```python
from build123d import *

# Parameters (mm, degrees)
BOSS_EXTRUDE1_DEPTH = 20
SKETCH3_R           = 2.5
CUT_EXTRUDE1_DEPTH  = 101.912910248
SKETCH4_R           = 2.5
BOSS_EXTRUDE2_DEPTH = 5
SKETCH5_R           = 2.25
CUT_EXTRUDE2_DEPTH  = 101.912910248
FILLET2_R           = 2


with BuildPart() as part:
    # Sketch2 → Boss-Extrude1 (new body)
    with BuildSketch(Plane(origin=(0, 0, 0), x_dir=(1, 0, 0), z_dir=(0, 1, 0))):
        with BuildLine():
            Line((-31.365303949, 0), (78.634696051, 0))
            add(Edge.make_bspline(
                [(-31.365303949, 60), (-8.421867165, 19.05257491), (40.3762891, 8.008963313), (78.634696051, 0)],
                knots=[0, 0, 0, 0, 1, 1, 1, 1], degree=3))
            Line((-31.365303949, 60), (-31.365303949, 0))
        make_face()
    extrude(amount=BOSS_EXTRUDE1_DEPTH)

    # Sketch3 → Cut-Extrude1 (cut, through all)
    with BuildSketch(Plane.XY):
        with Locations((-11.365303949, 10)):
            Circle(SKETCH3_R)
        with Locations((8.634696051, 10)):
            Circle(SKETCH3_R)
        with Locations((28.634696051, 10)):
            Circle(SKETCH3_R)
        with Locations((48.634696051, 10)):
            Circle(SKETCH3_R)
    extrude(amount=-CUT_EXTRUDE1_DEPTH, mode=Mode.SUBTRACT)

    # Sketch4 → Boss-Extrude2 (add)
    with BuildSketch(Plane.XY):
        with Locations((-11.365303949, 10)):
            Circle(SKETCH4_R)
        with Locations((8.634696051, 10)):
            Circle(SKETCH4_R)
        with Locations((28.634696051, 10)):
            Circle(SKETCH4_R)
        with Locations((48.634696051, 10)):
            Circle(SKETCH4_R)
    extrude(amount=-BOSS_EXTRUDE2_DEPTH)

    # Sketch5 → Cut-Extrude2 (cut, through all)
    with BuildSketch(Plane.XY):
        with Locations((-11.365303949, 10)):
            Circle(SKETCH5_R)
        with Locations((8.634696051, 10)):
            Circle(SKETCH5_R)
        with Locations((28.634696051, 10)):
            Circle(SKETCH5_R)
        with Locations((48.634696051, 10)):
            Circle(SKETCH5_R)
    extrude(amount=-CUT_EXTRUDE2_DEPTH, mode=Mode.SUBTRACT)

    # Fillet2
    fillet2_edges = [part.edges().sort_by_distance(p)[0] for p in [
        (16.640660288, 20, -18.214380109),
        (16.640660288, 0, -18.214380109),
    ]]
    fillet(fillet2_edges, radius=FILLET2_R)


solid = part.part
```
Source: CAD feature listing. Evaluate the final solid. Frame: model axes, mm. A direction names the side the tool comes from. Coordinates: 2 decimals unless noted, no trailing zeros. One line per item, written item: value.
1) Reachability of faces 1 (the face through (26.137, 10.11, -9.548)), 2 (the face through (-13.024, 11.521, -2.465)) from +Z, -Z, +X, -X, +Y, -Y: full face, straight path, thin tool, end or side. Return the list, or none.
Computed values:
face 1: -Z
face 2: +Z, -Z
2) Contact query for flat-ended pins moving along their axis: pin 1 (8 mm diameter, centred on x = 53.5, y = 12.5, fed in from -Z); pin 2 (6 mm diameter, centred on x = 48.63, y = 10, fed in from -Z); pin 3 (5 mm diameter, centred on y = 8.5, z = -36, fed in from +X). Output: stop coordinate, or through.
Computed values:
pin 1: stops at z = -6.73
pin 2: stops at z = -7.8
pin 3: stops at x = -8.67
3) Ray query, line 1 (X direction, y = 10, z = -25.5); line 2 (Z direction, x = -22, y = 15); line 3 (Z direction, x = 35.5, y = 4). Return the intervals inside material, ascending. Write a range as [from, to].
Computed values:
line 1: x = [-31.37, -13.87], [-8.87, 2.83]
line 2: z = [-46.44, 0]
line 3: z = [-10.89, 0]
4) Mould query, pull axis X, two halves, no side actions, for faces 3 (the face through (-13.863, 10.11, -21.242)), 4 (the face through (-4, 0, -12)), 5 (the face through (-31.365, 10, -30)), 6 (the face through (6.976, 11.521, -2.465)). Classes: released by +X, released by -X, zero draft, split by the parting line, or undercut.
Computed values:
face 3: undercut
face 4: zero draft
face 5: released by -X
face 6: undercut
5) Cut plane A-A on y = 10. State how many separate pieces and enclosed holes the cut face has, plus the area to 3 significant figures.
Computed values:
separate pieces: 5
enclosed holes: 0
area: 1,760 mm^2
